from build123d import *

# Parameters (mm, degrees)
BOSS_EXTRUDE1_DEPTH        = 8
CUT_EXTRUDE1_DEPTH         = 283.696502476
CUT_EXTRUDE2_DEPTH         = 283.696502476
F_6_5_6_5_DIAMETER_HOLE2_D = 6.5
CUT_EXTRUDE3_REACH         = 284.697


with BuildPart() as part:
    # Sketch1 → Boss-Extrude1 (new body)
    with BuildSketch(Plane.XY.offset(8)):
        Polygon((-154.499999959, -218.249999957), (154.500000044, -218.249999957), (179.500000086, -193.249999916), (179.500000086, 193.249999916), (154.500000044, 218.249999957), (-154.499999959, 218.249999957), (-179.5, 193.249999916), (-179.5, -193.249999916), align=None)
    extrude(amount=-BOSS_EXTRUDE1_DEPTH)

    # Sketch2 → Cut-Extrude1 (cut, through all)
    with BuildSketch(Plane(origin=(0, 0, 0), x_dir=(-1, 0, 0), z_dir=(0, 0, -1))):
        with BuildLine():
            Line((-107.857864329, -153.249999987), (107.857864423, -153.249999987))
            ThreePointArc((107.857864423, -153.249999987), (111.684698748, -152.488795312), (114.928932237, -150.321067798))
            Line((114.928932237, -150.321067798), (129.071067861, -136.178932174))
            ThreePointArc((129.071067861, -136.178932174), (131.23879537, -132.934698692), (132.000000044, -129.107864376))
            Line((132.000000044, -129.107864376), (132.000000044, 129.107864376))
            ThreePointArc((132.000000044, 129.107864376), (131.23879537, 132.934698692), (129.071067861, 136.178932174))
            Line((129.071067861, 136.178932174), (114.928932237, 150.321067798))
            ThreePointArc((114.928932237, 150.321067798), (111.684698748, 152.488795312), (107.857864423, 153.249999987))
            Line((107.857864423, 153.249999987), (-107.857864329, 153.249999987))
            ThreePointArc((-107.857864329, 153.249999987), (-111.684698653, 152.488795312), (-114.928932143, 150.321067798))
            Line((-114.928932143, 150.321067798), (-129.071067767, 136.178932174))
            ThreePointArc((-129.071067767, 136.178932174), (-131.238795276, 132.934698692), (-131.999999949, 129.107864376))
            Line((-131.999999949, 129.107864376), (-131.999999949, -129.107864376))
            ThreePointArc((-131.999999949, -129.107864376), (-131.238795276, -132.934698692), (-129.071067767, -136.178932174))
            Line((-129.071067767, -136.178932174), (-114.928932143, -150.321067798))
            ThreePointArc((-114.928932143, -150.321067798), (-111.684698653, -152.488795312), (-107.857864329, -153.249999987))
        make_face()
    extrude(amount=-CUT_EXTRUDE1_DEPTH, mode=Mode.SUBTRACT)

    # Sketch3 → Cut-Extrude2 (cut, through all)
    with BuildSketch(Plane(origin=(0, 0, 0), x_dir=(-1, 0, 0), z_dir=(0, 0, -1))):
        with BuildLine():
            Line((134.249999927, -198.50000003), (124.249999986, -198.50000003))
            ThreePointArc((124.249999986, -198.50000003), (122.835786445, -199.085786459), (122.250000016, -200.5))
            Line((122.250000016, -200.5), (122.250000016, -209.5))
            ThreePointArc((122.250000016, -209.5), (122.835786436, -210.91421352), (124.249999956, -211.49999994))
            Line((124.249999956, -211.49999994), (134.249999956, -211.49999994))
            ThreePointArc((134.249999956, -211.49999994), (135.664213457, -210.914213528), (136.249999869, -209.500000027))
            Line((136.249999869, -209.500000027), (136.249999869, -200.499999973))
            ThreePointArc((136.249999869, -200.499999973), (135.664213448, -199.085786451), (134.249999927, -198.50000003))
        make_face()
    extrude(amount=-CUT_EXTRUDE2_DEPTH, mode=Mode.SUBTRACT)

    # Ø6.5 (6.5) Diameter Hole2 (through all)
    with Locations(Plane(origin=(0, 0, 0), x_dir=(-1, 0, 0), z_dir=(0, 0, -1))):
        with Locations((-153.5, -182.25), (153.5, -182.25), (-153.5, 182.25), (153.5, 182.25)):
            Hole(F_6_5_6_5_DIAMETER_HOLE2_D / 2)

    # Sketch8 → Cut-Extrude3 (cut, up to next)
    with BuildSketch(Plane.XY.offset(8), mode=Mode.PRIVATE) as cut_extrude3_sk1:
        with BuildLine():
            Line((-89, -196.249999957), (-145, -196.249999957))
            ThreePointArc((-145, -196.249999957), (-146.414213562, -196.835786395), (-147, -198.249999957))
            Line((-147, -198.249999957), (-147, -218.249999957))
            Line((-147, -218.249999957), (-87, -218.249999957))
            Line((-87, -218.249999957), (-87, -198.249999957))
            ThreePointArc((-87, -198.249999957), (-87.585786438, -196.835786395), (-89, -196.249999957))
        make_face()
    cut_extrude3_tool1 = extrude(cut_extrude3_sk1.sketch, amount=-CUT_EXTRUDE3_REACH, mode=Mode.PRIVATE) & part.part
    add(cut_extrude3_tool1.solids().sort_by_distance((-117, -207.263744, 8))[0], mode=Mode.SUBTRACT)


solid = part.part
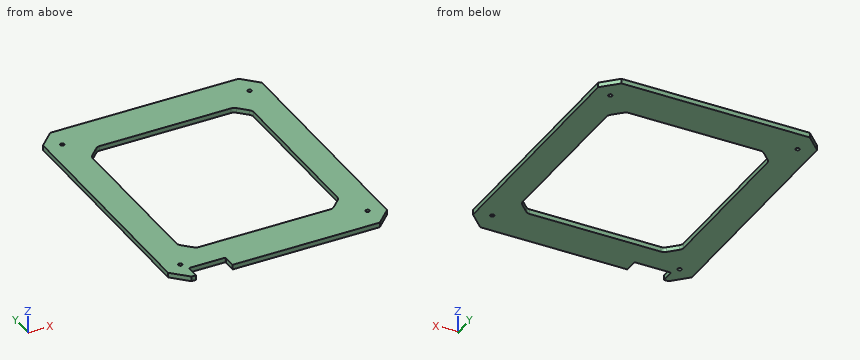
Input: part model. Units: mm. Frame: model coordinates. Coordinates: 2 decimals unless noted, no trailing zeros. Order: outer loops, then holes, each group sorted by start corner. A loop starts at its lowest first (then second) coordinate and runs counter-clockwise, first axis right, second up. Notation, with made-up numbers: M 14,87.5 L 31,87.5 A26 ccw 31,116.5 Z; hole C 71.5,65 d7. An arc over 180 degrees is marked long. Answer as CSV lines item,"result".
1. Section A-A (x = -19.5). Return the cut outline in (y, z), then the cut area to 3 significant figures.
Reported:
outline,"M -218.25,0 L -153.25,0 L -153.25,8 L -218.25,8 Z; M 153.25,0 L 218.25,0 L 218.25,8 L 153.25,8 Z"
area,"1,040 mm2"
2. Section B-B (y = 77.5). Return the cut outline in (x, z), then the cut area to 3 significant figures.
Reported:
outline,"M -179.5,0 L -132,0 L -132,8 L -179.5,8 Z; M 132,0 L 179.5,0 L 179.5,8 L 132,8 Z"
area,"760 mm2"
3. Section C-C (z = 5.75). State how many separate pieces and enclosed holes the cut face has, then the cut area to 3 significant figures.
Reported:
separate pieces,"1"
enclosed holes,"5"
area,"73,900 mm2"
4. Material intervals for line 1 (X direction, y = -182.25, z = 4.5); line 2 (Y direction, x = 153.5, z = 4.75); line 3 (X direction, y = -107, z = 7.75), sorted ascending. Write a range as from..to.
Reported:
line 1,"-179.5..-156.75, -150.25..150.25, 156.75..179.5"
line 2,"-218.25..-185.5, -179..179, 185.5..218.25"
line 3,"-179.5..-132, 132..179.5"
5. First-contact query: P1, Ø1.5, axis at x = -91.5, z = 2.5, coming from the -Y side; P2, Ø4, axis at y = -212.5, z = 4.5, coming from the +X side. Flat tips, straight axial feed; report the tip coordinate or a pass-through.
Reported:
P1,"y = -196.25"
P2,"x = 162.25"
